from build123d import *

# Parameters (mm, degrees)
F0_W      = 508
F0_H      = 508
F1_DEPTH  = 381
F2_W      = 495.299994
F2_H      = 495.299994
F3_DEPTH  = 374.65
F4_W      = 495.299994
F4_H      = 6.349997
F5_DEPTH  = 228.6
F6_W      = 193.675
F6_H      = 6.35
F7_DEPTH  = 228.6
F8_DEPTH  = 374.65
F6_W_2    = 295.274994
F6_H_2    = 6.350006
F9_DEPTH  = 374.65
F10_DEPTH = 50.8


with BuildPart() as f1:
    # F0 (on Top) → F1 (new body)
    with BuildSketch(Plane.XY):
        Rectangle(F0_W, F0_H)
    extrude(amount=F1_DEPTH)

    # F2 (on face) → F3 (cut)
    with BuildSketch(Plane.XY.offset(381)):
        Rectangle(F2_W, F2_H)
    extrude(amount=-F3_DEPTH, mode=Mode.SUBTRACT)

    # F4 (on face) → F5 (join)
    with BuildSketch(Plane.XY.offset(6.35)):
        with Locations((0, -92.074998)):
            Rectangle(F4_W, F4_H)
    extrude(amount=F5_DEPTH)

    # F6 (on face) → F7 (join)
    with BuildSketch(Plane.XY.offset(6.35)):
        with Locations((150.812497, -15.875003)):
            Rectangle(F6_W, F6_H)
    extrude(amount=F7_DEPTH)

    # F6 (on face) → F8 (join)
    with BuildSketch(Plane.XY.offset(6.35)):
        Polygon((53.974997, -12.700003), (53.974997, 247.649997), (47.624997, 247.649997), (47.624997, 146.050006), (47.624997, 139.7), (47.624997, -88.9), (53.974997, -88.9), (53.974997, -19.050003), align=None)
    extrude(amount=F8_DEPTH)

    # F6 (on face) → F9 (join)
    with BuildSketch(Plane.XY.offset(6.35)):
        with Locations((-100.0125, 142.875003)):
            Rectangle(F6_W_2, F6_H_2)
    extrude(amount=F9_DEPTH)

    # F6 (on face) → F10 (cut)
    with BuildSketch(Plane.XY.offset(6.35)):
        with Locations((150.812497, -15.875003)):
            Rectangle(F6_W, F6_H)
    extrude(amount=F10_DEPTH, mode=Mode.SUBTRACT)


solid = f1.part
Work out the finished part from the listing and answer in its coordinate system (mm). A direction names the side the tool comes from. Coordinates: 2 decimals unless noted, no trailing zeros. Write each loop counter-clockwise with the first axis right and the second up, starting at its lowest first coordinate (ties: lowest second). Pieces come first, ordered by that corner, then holes. Notation, with made-up numbers: M 21,10.25 L 39,10.25 A29 ccw 39,43.25 Z; hole C -36.75,10.25 d9. An arc over 180 degrees is marked long. Write item = value, one per line.
1. Flat-ended cylindrical pins translate along their axes: pin 1 (5 mm diameter, centred on x = -48.5, y = -92.5, fed in from +Z); pin 2 (4 mm diameter, centred on x = -24, y = 24, fed in from +Z). Find the tip coordinate at first contact, or state that the pin passes through.
Solution:
pin_1 = 234.95
pin_2 = 6.35
2. The part is cut by section C-C (z = 324). Determine the outline of the cut face in (x, y) (3 decimals).
Solution:
outline = M -254,-254 L 254,-254 L 254,254 L -254,254 Z; hole M -247.65,-247.65 L 247.65,-247.65 L 247.65,247.65 L 53.975,247.65 L 53.975,-88.9 L 47.625,-88.9 L 47.625,139.7 L -247.65,139.7 Z; hole M -247.65,146.05 L 47.625,146.05 L 47.625,247.65 L -247.65,247.65 Z
3. The part is cut by section D-D (y = -218). Determine the outline of the cut face in (x, z).
Solution:
outline = M -254,0 L 254,0 L 254,381 L 247.65,381 L 247.65,6.35 L -247.65,6.35 L -247.65,381 L -254,381 Z
4. The part is cut by section B-B (z = 103.5). Determine the outline of the cut face in (x, y) (3 decimals).
Solution:
outline = M -254,-254 L 254,-254 L 254,254 L -254,254 Z; hole M -247.65,-247.65 L 247.65,-247.65 L 247.65,-95.25 L -247.65,-95.25 Z; hole M -247.65,-88.9 L 47.625,-88.9 L 47.625,139.7 L -247.65,139.7 Z; hole M -247.65,146.05 L 47.625,146.05 L 47.625,247.65 L -247.65,247.65 Z; hole M 53.975,-88.9 L 247.65,-88.9 L 247.65,-19.05 L 53.975,-19.05 Z; hole M 53.975,-12.7 L 247.65,-12.7 L 247.65,247.65 L 53.975,247.65 Z
5. For faces 5 (the face through (-3, -95.25, 119)), 6 (the face through (-4, 254, 188)), determine the directions among +Z, -Z, +X, -X, +Y, -Y from which every point of the face is accessible in a straight line to the end or side of a thin tool.
Solution:
face_5 = +Z
face_6 = +Z, -Z, +X, -X, +Y
6. The part is cut by section A-A (x = 78.5). Determine the outline of the cut face in (y, z), then the cut area to 3 significant figures.
Solution:
outline = M -254,0 L 254,0 L 254,381 L 247.65,381 L 247.65,6.35 L -88.9,6.35 L -88.9,234.95 L -95.25,234.95 L -95.25,6.35 L -247.65,6.35 L -247.65,381 L -254,381 Z; M -19.05,57.15 L -12.7,57.15 L -12.7,234.95 L -19.05,234.95 Z
area = 10,600 mm2
7. Determine the mould class of faces 1 (the face through (-3, -170, 6.35)), 2 (the face through (254, -4, 188)), 3 (the face through (-4, 4, 0)), 4 (the face through (-254, -4, 188)) for opening direction X: released by +X, released by -X, zero draft, split by the parting line, or undercut.
Solution:
face_1 = undercut
face_2 = released by +X
face_3 = zero draft
face_4 = released by -X
8. Straight lines are drawn through the part: line 1 (Y direction, x = -162, z = 223); line 2 (X direction, y = -52.5, z = 229.5) (3 decimals); line 3 (Y direction, x = -136, z = 262). For each, find the intervals that lie inside material, in ascending order. Write a range as from..to.
Solution:
line_1 = -254..-247.65, -95.25..-88.9, 139.7..146.05, 247.65..254
line_2 = -254..-247.65, 47.625..53.975, 247.65..254
line_3 = -254..-247.65, 139.7..146.05, 247.65..254
